The figure shows three views and two pictorial views of one solid part (mm, origin at its lowest corner). Answer the questions. Round coordinates to 2 decimals unless told otherwise and drop trailing zeros. Order: outer loops, then holes, each group sorted by start corner. A loop starts at its lowest first (then second) coordinate and runs counter-clockwise, first axis right, second up. Notation, with made-up numbers: (-33.5, 63) -> (19.5, 63) arc R9 cw to (19.5, 72) -> close; hole circle Ø7 at (49.5, -16). An arc over 180 degrees is marked (long way). One line per item, written item: value. Start each with the question number.
1. The mould has two halves that part along X. Classify the marked faces 1, 2, 3 and 4: released by +X, released by -X, zero draft, split by the parting line, or undercut.
2. Section C-C (y = 13.75) is taken. Give the vertices of the cut face in (x, z), then the cut area to 3 significant figures.
3. Section A-A (x = 10) is taken. Give the vertices of the cut face in (y, z).
4. Consider line 1 (Y direction, x = 4.5, z = 10). Determine where the line is inside the solid, lowest interval first.
5. A flat-ended cylindrical pin translates along its axis: pin 1 Ø5 at (y, z) = (10, 10) entering from -X. Find the tip coordinate at first contact, or state that the pin passes through.
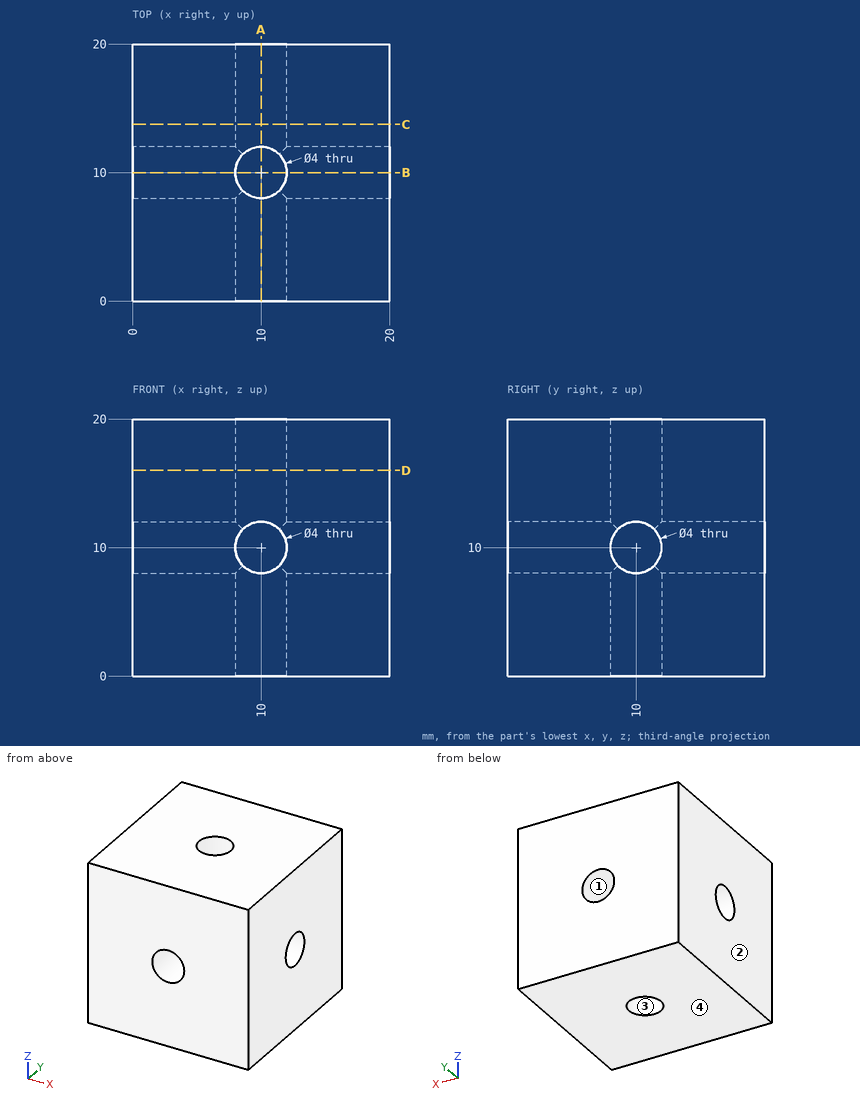
Answer:
1. face 1: undercut
1. face 2: released by -X
1. face 3: undercut
1. face 4: zero draft
2. outline: (0, 0) -> (20, 0) -> (20, 20) -> (0, 20) -> close; hole circle Ø4 at (10, 10)
2. area: 387 mm^2
3. outline: (0, 0) -> (8, 0) -> (8, 8) -> (0, 8) -> close; (0, 12) -> (8, 12) -> (8, 20) -> (0, 20) -> close; (12, 0) -> (20, 0) -> (20, 8) -> (12, 8) -> close; (12, 12) -> (20, 12) -> (20, 20) -> (12, 20) -> close
4. line 1: 0 to 8, 12 to 20
5. pin 1: x = 0
